from build123d import *

# Parameters (mm, degrees)
SKETCH1_W           = 50.55571166
SKETCH1_H           = 25.842581666
SKETCH1_R           = 2.249766629
SKETCH1_R_2         = 2.413
SKETCH1_W_2         = 22.225
SKETCH1_H_2         = 22.225
BOSS_EXTRUDE1_DEPTH = 3.175
FILLET1_R           = 2.54


with BuildPart() as part:
    # Sketch1 → Boss-Extrude1 (new body)
    with BuildSketch(Plane.XY):
        Rectangle(SKETCH1_W, SKETCH1_H)
        with Locations((17.4625, 0)):
            Circle(SKETCH1_R, mode=Mode.SUBTRACT)
        with Locations((-17.4625, 0)):
            Circle(SKETCH1_R_2, mode=Mode.SUBTRACT)
        Rectangle(SKETCH1_W_2, SKETCH1_H_2, mode=Mode.SUBTRACT)
    extrude(amount=BOSS_EXTRUDE1_DEPTH)

    # Fillet1
    fillet1_edges = [part.edges().sort_by_distance(p)[0] for p in [
        (-25.27785583, -12.921290833, 1.5875),
        (-25.27785583, 12.921290833, 1.5875),
        (25.27785583, 12.921290833, 1.5875),
        (25.27785583, -12.921290833, 1.5875),
    ]]
    fillet(fillet1_edges, radius=FILLET1_R)


solid = part.part
Check sheet for the modelled part. Datum: model origin and axes. Units: mm. A direction names the side the tool comes from. Round coordinates to 2 decimals unless told otherwise and drop trailing zeros. Loops run counter-clockwise (first coordinate to the right, second up) from the corner with the lowest first, then second, coordinate; pieces in that order, holes last.
1. Scan lines: probe 1 along X at (y, z) = (4, 0.6); probe 2 along X at (y, z) = (1.25, 0.6); probe 3 along Y at (x, z) = (-7.5, 1.65). Record each from-to range of solid material in increasing order.
2. Sectioned sample at D-D on x = -18.5. Record the boundary of the cut face in (y, z) (3 decimals).
3. Set-up check for faces 1 (the flat face through (-12, 0, 0)), 2 (the flat face through (-11.112, 0, 2)): record each of +Z, -Z, +X, -X, +Y, -Y from which the full face is reachable in a straight line by a thin tool's end or side.
4. Sectioned sample at B-B on y = 0. Record the boundary of the cut face in (x, z) (1 decimal).
5. Mould release check, pull along X, two halves, no side actions. Record for faces 3 (the flat face through (11.112, 0, 2)), 4 (the flat face through (-25.278, 0, 2)), 5 (the flat face through (0, 11.112, 2)), 6 (the flat face through (0, 12.921, 2)): released by +X, released by -X, zero draft, split by the parting line, or undercut.
6. Sectioned sample at C-C on z = 1.95. Record the boundary of the cut face in (x, y), and give its area (3 significant figures).
7. Gauge pin test, flat end, axial feed: pin 1 Ø3 at (x, y) = (19.5, 6.5) entering from -Z. Record the tip position at first contact, or that the pin passes through.
8. Sectioned sample at A-A on y = 4.5. Record the boundary of the cut face in (x, z) (1 decimal), and give its area (4 significant figures).
Recorded:
1. probe 1: x = -25.28 to -11.11, 11.11 to 25.28
1. probe 2: x = -25.28 to -19.53, -15.4 to -11.11, 11.11 to 15.59, 19.33 to 25.28
1. probe 3: y = -12.92 to -11.11, 11.11 to 12.92
2. outline: (-12.921, 0) - (-2.179, 0) - (-2.179, 3.175) - (-12.921, 3.175) - close; (2.179, 0) - (12.921, 0) - (12.921, 3.175) - (2.179, 3.175) - close
3. face 1: -Z, +X, -X, +Y, -Y
3. face 2: +Z, -Z
4. outline: (-25.3, 0) - (-19.9, 0) - (-19.9, 3.2) - (-25.3, 3.2) - close; (-15, 0) - (-11.1, 0) - (-11.1, 3.2) - (-15, 3.2) - close; (11.1, 0) - (15.2, 0) - (15.2, 3.2) - (11.1, 3.2) - close; (19.7, 0) - (25.3, 0) - (25.3, 3.2) - (19.7, 3.2) - close
5. face 3: undercut
5. face 4: released by -X
5. face 5: undercut
5. face 6: zero draft
6. outline: (-25.28, -10.38) arc R2.54 ccw to (-22.74, -12.92) - (22.74, -12.92) arc R2.54 ccw to (25.28, -10.38) - (25.28, 10.38) arc R2.54 ccw to (22.74, 12.92) - (-22.74, 12.92) arc R2.54 ccw to (-25.28, 10.38) - close; hole circle Ø4.83 at (-17.46, 0); hole (-11.11, -11.11) - (11.11, -11.11) - (11.11, 11.11) - (-11.11, 11.11) - close; hole circle Ø4.5 at (17.46, 0)
6. area: 773 mm2
7. pin 1: stops at z = 0
8. outline: (-25.3, 0) - (-11.1, 0) - (-11.1, 3.2) - (-25.3, 3.2) - close; (11.1, 0) - (25.3, 0) - (25.3, 3.2) - (11.1, 3.2) - close
8. area: 89.95 mm2
